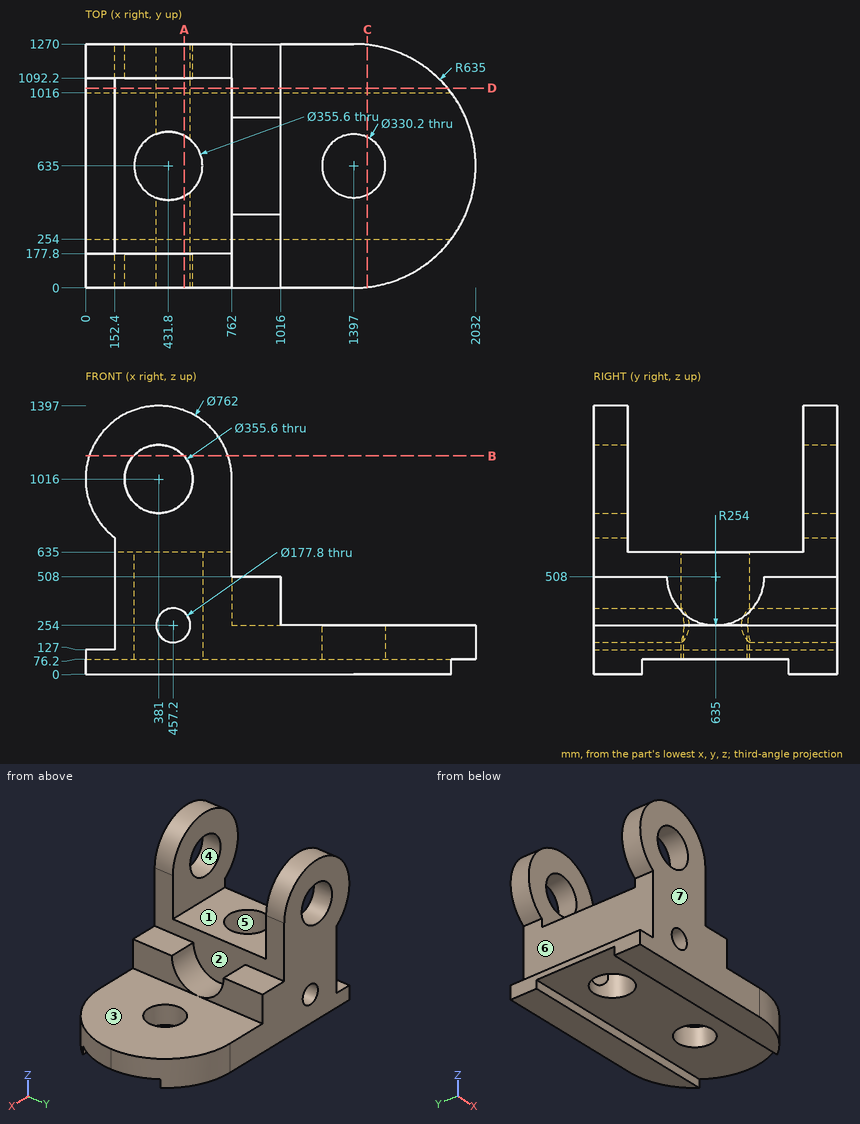
Could you check a few things on this drawing? It's one solid part, dimensions in mm from its lowest x, y, z. A direction names the side the tool comes from. Give positions to 0.01 mm unless a question says otherwise; leave off trailing zeros. Order: outer loops, then holes, each group sorted by start corner. A loop starts at its lowest first (then second) coordinate and runs counter-clockwise, first axis right, second up. Notation, with made-up numbers: M 18.5,-38.5 L 37.5,-38.5 A23 ccw 37.5,0.5 Z; hole C 6.5,47 d11. An arc over 180 degrees is marked long. Use one line per item in the form item = value.
Item 1: If I drill on line 1 along X through (y, z) = (108, 1016); line 2 along Y through (x, z) = (233, 696); line 3 along Y through (x, z) = (431.8, 499.5), over which ranges is the centre line in solid material (lowest first)? Write a range as [from, to].
Values follow:
line_1 = [0, 203.2], [558.8, 762]
line_2 = [0, 177.8], [1092.2, 1270]
line_3 = [0, 457.2], [812.8, 1270]
Item 2: If we section it at C-C, the plane x = 1467.5: Write out the boundary of the cut face in (y, z), and give its area (3 significant figures).
Values follow:
outline = M 3.93,0 L 254,0 L 254,76.2 L 485.71,76.2 L 485.71,254 L 3.93,254 Z; M 784.29,76.2 L 1016,76.2 L 1016,0 L 1266.07,0 L 1266.07,254 L 784.29,254 Z
area = 209,000 mm^2
Item 3: If we section it at B-B, the plane z = 1136: Write out the boundary of the cut face in (x, y), and give its area (3 significant figures).
Values follow:
outline = M 19.39,0 L 249.8,0 L 249.8,177.8 L 19.39,177.8 Z; M 19.39,1092.2 L 249.8,1092.2 L 249.8,1270 L 19.39,1270 Z; M 512.2,0 L 742.61,0 L 742.61,177.8 L 512.2,177.8 Z; M 512.2,1092.2 L 742.61,1092.2 L 742.61,1270 L 512.2,1270 Z
area = 164,000 mm^2
Item 4: Thinking about a two-plate mould opening in X: for the marked faces 4, 5, 6 and 7, which applies, pulls with the +X half, pulls with the -X half, needs draft (parallel to the pull), parting line crosses it, or undercut?
Values follow:
face_4 = undercut
face_5 = undercut
face_6 = pulls with the -X half
face_7 = needs draft
Item 5: For the marked faces 1, 2 and 3, which set-ups out of +Z, -Z, +X, -X, +Y, -Y let a thin tool reach every point of the face, with its end or its side?
Values follow:
face_1 = +Z, +X, -X
face_2 = +Z, +X
face_3 = +Z, +X, +Y, -Y
Item 6: If we section it at A-A, the plane x = 515: Count the separate pieces of the cut face and the enclosed holes in it, and give its area (3 significant figures).
Values follow:
separate_pieces = 6
enclosed_holes = 0
area = 623,000 mm^2
Item 7: If we section it at D-D, the plane y = 1040: Write out the boundary of the cut face in (x, z), and give its area (3 significant figures).
Values follow:
outline = M 0,0 L 1886.08,0 L 1886.08,254 L 1016,254 L 1016,508 L 762,508 L 762,635 L 152.4,635 L 152.4,127 L 0,127 Z; hole C 457.2,254 d177.8
area = 732,000 mm^2
Item 8: Will these pins go through, and if not, where does the flat tip stop? pin 1 Ø6 at (x, y) = (691.5, 143) entering from +Z (3 decimals); pin 2 Ø1 at (x, y) = (1675.5, 246.5) entering from +Z; pin 3 Ø2 at (x, y) = (1594.5, 311.5) entering from -Z.
Values follow:
pin_1 = 1240.955
pin_2 = 254
pin_3 = 76.2
